```python
from build123d import *

# Parameters (mm, degrees)
F1_DEPTH = 25.4
F3_DEPTH = 6.35
F5_DEPTH = 6.35


with BuildPart() as f1:
    # F0 (on Front) → F1 (new body)
    with BuildSketch(Plane.XZ):
        Polygon((37.471404, 31.743777), (0, 31.743777), (0, 0), (38.1, 0), align=None)
    extrude(amount=F1_DEPTH)

    # F2 (on face) → F3 (cut)
    with BuildSketch(Plane.XZ.offset(25.4)):
        Polygon((37.471404, 31.743777), (12.7, 31.743777), (12.7, 0), (38.1, 0), align=None)
    extrude(amount=-F3_DEPTH, mode=Mode.SUBTRACT)

    # F4 (on face) → F5 (cut)
    with BuildSketch(Plane(origin=(0, 0, 0), x_dir=(-1, 0, 0), z_dir=(0, 1, 0))):
        Polygon((-38.1, 0), (-12.7, 0), (-12.7, 8.530987), (-12.7, 31.743777), (-37.471404, 31.743777), align=None)
    extrude(amount=-F5_DEPTH, mode=Mode.SUBTRACT)


solid = f1.part
```
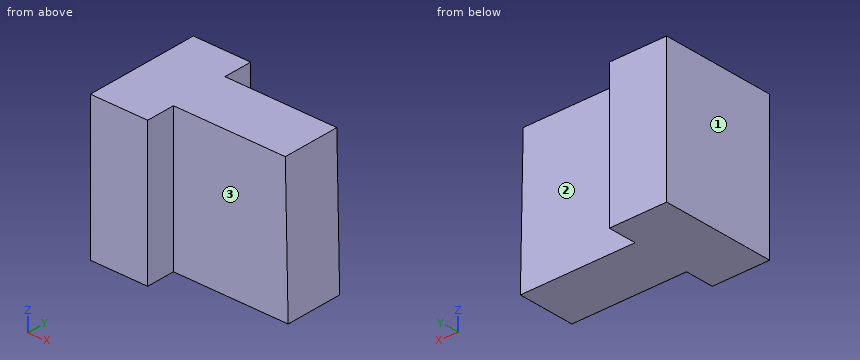
Check sheet for the modelled part. Datum: model origin and axes. Units: mm. Face numbers are marked on the shaded views. A direction names the side the tool comes from. Give positions to 0.01 mm unless a question says otherwise; leave off trailing zeros. Write each loop counter-clockwise with the first axis right and the second up, starting at its lowest first coordinate (ties: lowest second). Pieces come first, ordered by that corner, then holes. Notation, with made-up numbers: (36.25, 58) - (58.25, 58) arc R6 cw to (58.25, 67) - close; hole circle Ø9 at (-4.75, -19). An arc over 180 degrees is marked (long way). Answer as a JSON object with one key per item and string values. Group by question number.
1) Sectioned sample at A-A (z = 8.5). Record the cut outline in (x, y), then the cut area to 3 significant figures.
2) Access from +Z, -Z, +X, -X, +Y, -Y to the whole of each face (thin tool, end or side, straight path). Record for the marked faces 1, 2 and 3.
3) Depth check by flat-ended pin: P1, Ø3, axis at x = 22.5, y = -21, coming from the -Z side; P2, Ø4, axis at x = 15.5, z = 8, coming from the -Y side; P3, Ø12.5, axis at x = 27, z = 11.5, coming from the +Y side; P4, Ø1.9, axis at y = -23, z = 22, coming from the +X side. Enter the tip coordinate at first touch or a pass-through.
4) Thickness scan on probe 1 along X at (y, z) = (-6.25, 21.5); probe 2 along Y at (x, z) = (32, 28.5); probe 3 along X at (y, z) = (-11.75, 18). Record the ranges inside material, lowest first. Write a range as from..to.
5) Sectioned sample at B-B (y = -22). Record the cut outline in (x, z).
6) Sectioned sample at D-D (z = 3). Record the cut outline in (x, y), then the cut area to 3 significant figures.
7) Sectioned sample at C-C (x = 35). Record the cut outline in (y, z).
Geometry results:
{
 "1": {"outline": "(0, -25.4) - (12.7, -25.4) - (12.7, -19.05) - (37.93, -19.05) - (37.93, -6.35) - (12.7, -6.35) - (12.7, 0) - (0, 0) - close", "area": "643 mm^2"},
 "2": {"face 1": "+Z, -Z, -X, +Y, -Y", "face 2": "+Z, -Z, +X, +Y", "face 3": "+Z, -Z, +X, -Y"},
 "3": {"P1": "passes through", "P2": "stops at y = -19.05", "P3": "stops at y = -6.35", "P4": "stops at x = 12.7"},
 "4": {"probe 1": "x = 0..12.7", "probe 2": "y = -19.05..-6.35", "probe 3": "x = 0..37.74"},
 "5": {"outline": "(0, 0) - (12.7, 0) - (12.7, 31.74) - (0, 31.74) - close"},
 "6": {"outline": "(0, -25.4) - (12.7, -25.4) - (12.7, -19.05) - (38.04, -19.05) - (38.04, -6.35) - (12.7, -6.35) - (12.7, 0) - (0, 0) - close", "area": "644 mm^2"},
 "7": {"outline": "(-19.05, 0) - (-6.35, 0) - (-6.35, 31.74) - (-19.05, 31.74) - close"}
}
